Can you work these out from the model? Positions are in its coordinate system, mm. Face numbers are marked on the shaded views. Give positions to 0.01 mm unless a question says otherwise; leave off trailing zeros. Write each loop counter-clockwise with the first axis right and the second up, starting at its lowest first coordinate (ties: lowest second). Pieces come first, ordered by that corner, then holes.
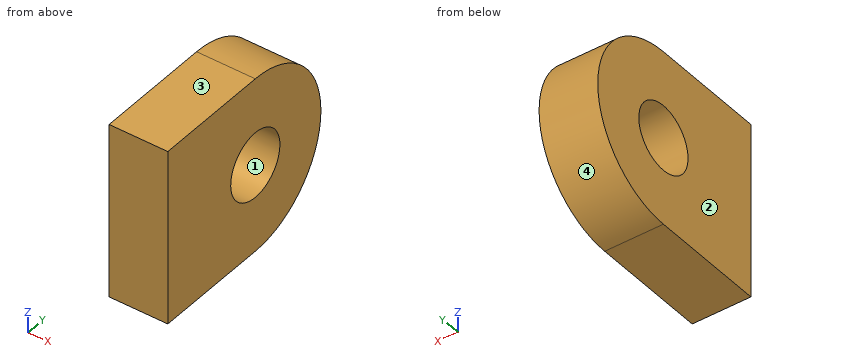
from build123d import *

# Parameters (mm, degrees)
SKETCH1_R           = 14.2875
BOSS_EXTRUDE1_DEPTH = 12.7


with BuildPart() as part:
    # Sketch1 → Boss-Extrude1 (new body, symmetric)
    with BuildSketch(Plane(origin=(0, 0, 0), x_dir=(0, 0, -1), z_dir=(1, 0, 0))):
        with BuildLine():
            Line((-38.1, 0), (38.1, 0))
            Line((38.1, 0), (38.1, 50.8))
            ThreePointArc((38.1, 50.8), (0, 88.9), (-38.1, 50.8))
            Line((-38.1, 50.8), (-38.1, 0))
        make_face()
        with Locations((0, 50.8)):
            Circle(SKETCH1_R, mode=Mode.SUBTRACT)
    extrude(amount=BOSS_EXTRUDE1_DEPTH, both=True)


solid = part.part
(1) If we mould it in two halves opening along Z, with no side actions, what happens to the marked faces 1, 2, 3 and 4? For each: +Z half, -Z half, draft (parallel to the pull), parting line (faces both ways), or undercut.
Returned:
face 1: undercut
face 2: draft
face 3: +Z half
face 4: parting line
(2) Imagine slicing it at C-C, the plane y = 62. Write out the boundary of the cut face in (x, z).
Returned:
outline: (-12.7, -36.42) - (12.7, -36.42) - (12.7, -8.87) - (-12.7, -8.87) - close; (-12.7, 8.87) - (12.7, 8.87) - (12.7, 36.42) - (-12.7, 36.42) - close
(3) Will this pin go through, and if not, where does the flat tip stop? P1, Ø10, axis at x = 9, z = 11.5, coming from the +Y side.
Returned:
P1: stops at y = 88.34
(4) Imagine slicing it at B-B, the plane x = -5.5. Write out the boundary of the cut face in (y, z) (1 decimal), plus the area to 3 significant figures.
Returned:
outline: (0, -38.1) - (50.8, -38.1) arc R38.1 ccw to (50.8, 38.1) - (0, 38.1) - close; hole circle Ø28.6 at (50.8, 0)
area: 5,510 mm2
(5) Imagine slicing it at A-A, the plane z = 0. Write out the boundary of the cut face in (x, y), plus the area to 3 significant figures.
Returned:
outline: (-12.7, 0) - (12.7, 0) - (12.7, 36.51) - (-12.7, 36.51) - close; (-12.7, 65.09) - (12.7, 65.09) - (12.7, 88.9) - (-12.7, 88.9) - close
area: 1,530 mm2
(6) Imagine slicing it at D-D, the plane z = -30. Write out the boundary of the cut face in (x, y).
Returned:
outline: (-12.7, 0) - (12.7, 0) - (12.7, 74.29) - (-12.7, 74.29) - close
(7) If I drill on L1, parallel to Z at x = 10, y = 50; L2, parallel to Y at x = -2.75, z = 0; L3, parallel to Z at x = 3.5, y = 57, over which ranges is the centre line in solid material (lowest first)?
Returned:
L1: z = -38.1 to -14.27, 14.27 to 38.1
L2: y = 0 to 36.51, 65.09 to 88.9
L3: z = -37.59 to -12.87, 12.87 to 37.59
